Solid Edge part; units mm, degrees
sketch "Sketch1" plane through (0, 0, 0) normal (0, -1, 0) x (1, 0, 0)
  line L0 (40.3582, 0) -> (0, 0)
  line L1 (0, 0) -> (0, 18.2807)
  line L2 (0, 18.2807) -> (40.3582, 18.2807)
  arc A0 (40.3582, 18.2808) -> (40.3582, 0) centre (40.3582, 9.1404) cw
extrude "Protrusion1" add sketch "Sketch1" against normal blind 17.4305
sketch "Sketch2" plane through (0, 0, 0) normal (0, -1, 0) x (1, 0, 0)
  circle A0 centre (29.7379, 18.2807) radius 7.1267
extrude "ExtrudedCutout_1" cut sketch "Sketch2" against normal blind 28.8602
sketch "Sketch3" plane through (24.7493, 0, 9.1404) normal (0, -1, 0) x (1, 0, 0)
  line L0 (-15.6782, 9.1404) -> (-15.6782, 0.3921)
  line L1 (-15.6782, 0.3921) -> (-24.7493, 0.3921)
  line L2 (-24.7493, 0.3921) -> (-24.7493, 9.1404)
  line L3 (-24.7493, 9.1404) -> (-15.6782, 9.1404)
extrude "ExtrudedCutout_2" cut sketch "Sketch3" against normal blind 8.6187
Input: part model. Units: mm. Frame: model coordinates. A direction names the side the tool comes from. Coordinates: 2 decimals unless noted, no trailing zeros. Loops run counter-clockwise (first coordinate to the right, second up) from the corner with the lowest first, then second, coordinate; pieces in that order, holes last.
Q1. Cut plane A-A (z = 16.75). Output: boundary loops of the cut face in (x, y).
Q2. Draft query along X for faces 1 (the face through (9.071, 4, 14)), 2 (the face through (25, 0, 7)), 3 (the face through (29.581, 8.593, 11.156)). Return one class per face: +X half, -X half, draft (parallel to the pull), parting line (faces both ways), or undercut.
Q3. Cut plane C-C (x = 3.5). Output: boundary loops of the cut face in (y, z).
Q4. Material intervals for line 1 (Z direction, x = 6, y = 4); line 2 (X direction, y = 0.5, z = 15.25); line 3 (X direction, y = 16, z = 11.75), sorted ascending.
Q5. Set-up query: faces 4 (the face through (25, 17.43, 9)), 5 (the face through (5, 4, 9.532)). Return all of +Z, -Z, +X, -X, +Y, -Y with unobstructed straight access to the full face (end or side cutting, diameter ignored); none if empty.
Q6. Contact query for flat-ended pins moving along their axis: pin 1 (4 mm diameter, centred on x = 29, y = 14, fed in from +Z); pin 2 (1 mm diameter, centred on y = 7, z = 7.5, fed in from +X); pin 3 (9.5 mm diameter, centred on y = 3.5, z = 15.5, fed in from -X). Output: stop coordinate, or through.
Working result:
1. outline: (0, 8.62) - (9.07, 8.62) - (9.07, 0) - (22.78, 0) - (22.78, 17.43) - (0, 17.43) - close; (36.7, 0) - (45.42, 0) - (45.42, 17.43) - (36.7, 17.43) - close
2. face 1: -X half
2. face 2: draft
2. face 3: undercut
3. outline: (0, 0) - (17.43, 0) - (17.43, 18.28) - (8.62, 18.28) - (8.62, 9.53) - (0, 9.53) - close
4. line 1: z = 0 to 9.53
4. line 2: x = 9.07 to 23.29, 36.19 to 47.16
4. line 3: x = 0 to 26.88, 32.59 to 49.12
5. face 4: +Z, -Z, +X, -X, +Y
5. face 5: +Z, -X, -Y
6. pin 1: stops at z = 11.7
6. pin 2: stops at x = 49.43
6. pin 3: stops at x = 9.07
